Here's how the part is built. I have some questions about the finished solid (model axes, mm). Round coordinates to 2 decimals unless told otherwise and drop trailing zeros. Loops run counter-clockwise (first coordinate to the right, second up) from the corner with the lowest first, then second, coordinate; pieces in that order, holes last. Notation, with made-up numbers: M 82,61.25 L 136,61.25 A22 cw 136,74.25 Z; hole C 26.25,76.25 d11. An arc over 180 degrees is marked long. Answer as a JSON object with one key per item and string values.
from build123d import *

# Parameters (mm, degrees)
F0_W     = 80
F0_H     = 80
F0_R     = 1.5
F1_DEPTH = 3.175
F2_R     = 1.5
F3_DEPTH = 25


with BuildPart() as f1:
    # F0 (on Top) → F1 (new body)
    with BuildSketch(Plane.XY):
        Rectangle(F0_W, F0_H)
        with Locations((-22.722, -23.282524)):
            Circle(F0_R, mode=Mode.SUBTRACT)
        with Locations((22.822, -22.822)):
            Circle(F0_R, mode=Mode.SUBTRACT)
        with Locations((-23.182524, 22.261476)):
            Circle(F0_R, mode=Mode.SUBTRACT)
        with Locations((22.361476, 22.722)):
            Circle(F0_R, mode=Mode.SUBTRACT)
    extrude(amount=F1_DEPTH)

    # F2 (on face) → F3 (cut)
    with BuildSketch(Plane.XY.offset(3.175)):
        with Locations((-12.5, 12.5)):
            Circle(F2_R)
        with Locations((12.5, 12.5)):
            Circle(F2_R)
        with Locations((12.5, -12.5)):
            Circle(F2_R)
        with Locations((-12.5, -12.5)):
            Circle(F2_R)
    extrude(amount=-F3_DEPTH, mode=Mode.SUBTRACT)


solid = f1.part
Item 1: I want a section at A-A on y = 12.5. List the corners of the cut face in (x, z) for me (3 decimals), plus the area to 3 significant figures.
Solution:
{"outline": "M -40,0 L -14,0 L -14,3.175 L -40,3.175 Z; M -11,0 L 11,0 L 11,3.175 L -11,3.175 Z; M 14,0 L 40,0 L 40,3.175 L 14,3.175 Z", "area": "235 mm2"}
Item 2: If I drill on L1, parallel to Y at x = -12.5, z = 1.55; L2, parallel to X at y = 23.5, z = 0.45; L3, parallel to Y at x = -21.5, z = 0.95, over which ranges is the centre line in solid material (lowest first)? Write a range as from..to.
Solution:
{"L1": "y = -40..-14, -11..11, 14..40", "L2": "x = -40..-24.03, -22.34..21.08, 23.64..40", "L3": "y = -40..-24.15, -22.41..40"}
Item 3: We'd pull the mould along Y, two halves only. Please class faces 1 (the face through (-1, -40, 2)), 2 (the face through (-24.68, 22.33, 1.57)), 3 (the face through (-1, 40, 2)), 4 (the face through (-40, -1, 2)): +Y half, -Y half, draft (parallel to the pull), parting line (faces both ways), or undercut.
Solution:
{"face 1": "-Y half", "face 2": "undercut", "face 3": "+Y half", "face 4": "draft"}
